Work out the finished part from the listing and answer in its coordinate system (mm). A direction names the side the tool comes from. Round coordinates to 2 decimals unless told otherwise and drop trailing zeros. Order: outer loops, then holes, each group sorted by start corner. A loop starts at its lowest first (then second) coordinate and runs counter-clockwise, first axis right, second up. Notation, with made-up numbers: (68, -18.75) - (72, -18.75) arc R26 ccw to (72, -3.75) - close; hole circle Ø3 at (38, 50). An arc over 180 degrees is marked (long way). Answer in a Markdown table with one row per item.
Autodesk Inventor part; units mm, degrees
ref_plane "Arbeitsebene2" through (4.7579, -7.132, 2.2) normal (0, 0, 1) x (1, 0, 0)
ref_plane "YZ Plane" through (0, 0, 0) normal (1, 0, 0) x (0, 1, 0)
ref_plane "XZ Plane" through (0, 0, 0) normal (0, 1, 0) x (-1, 0, 0)
ref_plane "Arbeitsebene1" through (0, 0, 0) normal (0, 0, 1) x (1, 0, 0)
sketch "Skizze1" plane through (0, 0, 0) normal (0, 0, 1) x (1, 0, 0)
  circle A0 centre (-0.0001, 0.0021) radius 3
  circle A1 centre (11, 0) radius 2.566
  circle A2 centre (-9.5, -11) radius 1.352
  arc A3 (19, -13.5) -> (20, -12.5) centre (19, -12.5) ccw
  line L0 (20, -12.5) -> (20, 12.5)
  arc A4 (20, 12.5) -> (19, 13.5) centre (19, 12.5) ccw
  line L1 (19, 13.5) -> (-19, 13.5)
  arc A5 (-19, 13.5) -> (-20, 12.5) centre (-19, 12.5) ccw
  line L2 (-20, 12.5) -> (-20, -12.5)
  arc A6 (-20, -12.5) -> (-19, -13.5) centre (-19, -12.5) ccw
  line L3 (-19, -13.5) -> (19, -13.5)
  line L4 (18.6579, -7.132) -> (11.0758, -7.132)
  line L5 (18.6579, -7.132) -> (18.6579, 2.268)
  line L6 (18.6579, 2.268) -> (19.6579, 4.268)
  line L7 (19.6579, 4.268) -> (19.6579, 7.668)
  line L8 (18.0704, 7.668) -> (19.6579, 7.668)
  line L9 (18.0704, 7.668) -> (18.0704, 6.818)
  line L10 (18.0704, 6.818) -> (13.4704, 6.818)
  line L11 (13.4704, 6.818) -> (13.4704, 5.418)
  line L12 (13.4704, 5.418) -> (14.8704, 5.418)
  line L13 (14.8704, 5.418) -> (15.4704, 6.018)
  line L14 (15.4704, 6.018) -> (18.0704, 6.018)
  line L15 (18.0704, 6.018) -> (18.0704, 5.768)
  line L16 (18.0704, 5.768) -> (15.5704, 5.768)
  line L17 (15.5704, 5.768) -> (15.0704, 5.268)
  line L18 (15.0704, 5.268) -> (13.0704, 5.268)
  line L19 (13.0704, 5.268) -> (13.0704, 7.668)
  line L20 (6.4079, 7.668) -> (13.0704, 7.668)
  line L21 (6.4079, 7.668) -> (6.4079, 6.468)
  line L22 (4.7579, 6.468) -> (6.4079, 6.468)
  line L23 (4.7579, -7.132) -> (4.7579, 6.468)
  line L24 (5.4458, -7.132) -> (4.7579, -7.132)
  line L25 (5.4458, -7.132) -> (5.4458, -6.382)
  line L26 (5.4458, -6.382) -> (11.0758, -6.382)
  line L27 (11.0758, -6.382) -> (11.0758, -7.132)
  line L28 (9.0327, 10.168) -> (-5.2421, 10.168)
  line L29 (-5.2421, 10.168) -> (-5.2421, 8.168)
  line L30 (-5.2421, 8.168) -> (9.0327, 8.168)
  line L31 (9.0327, 8.168) -> (9.0327, 10.168)
  line L32 (-5.2421, 8.168) -> (4.7579, 8.168)
  line L33 (4.7579, 8.168) -> (4.7579, -9.632)
  line L34 (4.7579, -9.632) -> (-5.2421, -9.632)
  line L35 (-5.2421, -9.632) -> (-5.2421, 8.168)
  line L36 (4.7579, -9.632) -> (9.0327, -9.632)
  line L37 (9.0327, -9.632) -> (9.0327, -7.632)
  line L38 (9.0327, -7.632) -> (4.7579, -7.632)
  line L39 (4.7579, -7.632) -> (4.7579, -9.632)
  point P0 (0, 0)
  point P1 (4.7579, 8.168)
  dimension "d0" = 0
  dimension "d1" = 0.5
  dimension "d2" = 0.5
  dimension "d3" = 2
  dimension "d4" = 2
  dimension "d5" = 10
ref_plane "Arbeitsebene2" through (4.7579, -7.132, 2.2) normal (0, 0, 1) x (1, 0, 0)
extrude "Extrusion1" add sketch "Skizze1" along normal up to surface (2.2 mm away) contours A0 | L33 L34 L35 L30 L23 | L38 L37 L36 L33 | L30 L29 L28 L31
sketch "Skizze2" plane through (-5.2421, 10.168, 2.2) normal (0, 0, 1) x (1, 0, 0)
  line L0 (0, 0) -> (14.2747, 0)
  line L1 (0, -19.8) -> (0, 0)
  line L2 (14.2747, -19.8) -> (0, -19.8)
  line L3 (14.2747, -17.8) -> (14.2747, -19.8)
  line L4 (10, -17.8) -> (14.2747, -17.8)
  line L5 (10, -2) -> (10, -17.8)
  line L6 (14.2747, -2) -> (10, -2)
  line L7 (14.2747, 0) -> (14.2747, -2)
  line L8 (14.2747, 0) -> (0, 0)
  line L9 (14.2747, 0) -> (0, 0)
  line L10 (0, 0) -> (0, -19.8)
  line L11 (0, -19.8) -> (14.2747, -19.8)
  line L12 (14.2747, -19.8) -> (14.2747, 0)
  line L13 (9.6421, -14.568) -> (0.8421, -14.568)
  line L14 (0.8421, -14.568) -> (0.8421, -5.768)
  line L15 (0.8421, -5.768) -> (9.6421, -5.768)
  line L16 (9.6421, -5.768) -> (9.6421, -14.568)
  line L17 (9.6421, -14.568) -> (0.8421, -5.768) construction
  line L18 (0.8421, -14.568) -> (9.6421, -5.768) construction
  line L19 (0, 0) -> (0, -19.8)
  line L20 (0.8421, -5.768) -> (0, -5.768)
  line L21 (0, -5.768) -> (0, -14.568)
  line L22 (0, -14.568) -> (0.8421, -14.568)
  line L23 (0.8421, -14.568) -> (0.8421, -5.768)
  point P0 (5.2421, -10.168)
  point P1 (0, -5.768)
  point P2 (0.8421, -14.568)
  point P3 (14.2747, -17.8)
  point P4 (14.2747, -2)
  dimension "d8" = 8.8
  dimension "d9" = 8.8
extrude "Extrusion2" add sketch "Skizze2" along normal blind 2 contours L0 L7 L6 L5 L4 L3 L2 L1 L22 L13 L16 L15 L20 | L12 L4 L5 L6
sketch "Skizze3" plane through (0, 0, 0) normal (0, 0, -1) x (-1, 0, 0)
  line L0 (5.2421, 10.168) -> (5.2421, -9.632)
  line L1 (-9.0327, 10.168) -> (5.2421, 10.168)
  line L2 (-9.0327, 8.168) -> (-9.0327, 10.168)
  line L3 (-4.7579, 8.168) -> (-9.0327, 8.168)
  line L4 (-4.7579, -7.632) -> (-4.7579, 8.168)
  line L5 (-9.0327, -7.632) -> (-4.7579, -7.632)
  line L6 (-9.0327, -9.632) -> (-9.0327, -7.632)
  line L7 (5.2421, -9.632) -> (-9.0327, -9.632)
  line L8 (2.2421, -9.8367) -> (9.0217, -9.8367)
  line L9 (9.0217, -9.8367) -> (9.0217, 10.4786)
  line L10 (9.0217, 10.4786) -> (2.2421, 10.4786)
  line L11 (2.2421, 10.4786) -> (2.2421, -9.8367)
  line L12 (2.2421, -9.8367) -> (9.0217, 10.4786) construction
  line L13 (9.0217, -9.8367) -> (2.2421, 10.4786) construction
  point P0 (0, 0)
  point P1 (5.6319, 0.321)
  dimension "d12" = 3
extrude "Extrusion3" cut sketch "Skizze3" against normal blind 2.5 contours L1 L11 L10 L9 L8 L7 L0 | L0 L7 L11 L1
sketch "Skizze4" plane through (0, 0, 0) normal (0, 0, -1) x (-1, 0, 0)
  line L0 (2.2421, -9.632) -> (2.2421, 10.168)
  line L1 (-9.0327, 10.168) -> (2.2421, 10.168)
  line L2 (-9.0327, 8.168) -> (-9.0327, 10.168)
  line L3 (-4.7579, 8.168) -> (-9.0327, 8.168)
  line L4 (-4.7579, -7.632) -> (-4.7579, 8.168)
  line L5 (-9.0327, -7.632) -> (-4.7579, -7.632)
  line L6 (-9.0327, -9.632) -> (-9.0327, -7.632)
  line L7 (2.2421, -9.632) -> (-9.0327, -9.632)
  line L8 (2.2421, 4.4) -> (2.2421, 10.168)
  line L9 (2.2421, 9.168) -> (-1.1963, 9.168)
  line L10 (-1.1963, 9.168) -> (-1.1963, -8.632)
  line L11 (-1.1963, -8.632) -> (2.2421, -8.632)
  line L12 (2.2421, -8.632) -> (2.2421, 9.168)
  point P0 (0, 0)
  point P1 (2.2421, -8.632)
extrude "Extrusion4" cut sketch "Skizze4" against normal blind 2 contours L11 L10 L9 L0
equation "\"d6\" = d2"
properties part number "Anglerfish_Cameraspacer"
1) Find section D-D, the plane x = 5.5. Give the vertices of the cut face in (y, z).
Filled in:
| item | result |
|---|---|
| outline | (-9.63, 0) - (-7.63, 0) - (-7.63, 2.2) - (8.17, 2.2) - (8.17, 0) - (10.17, 0) - (10.17, 4.2) - (-9.63, 4.2) - close |
2) Find the intervals of material crossed by probe 1 along Y at (x, z) = (5.5, 1.65); probe 2 along Y at (x, z) = (-1.75, 1.9); probe 3 along Z at (x, y) = (-4.25, 8.75), in increasing order. Write a range as from..to.
Filled in:
| item | result |
|---|---|
| probe 1 | y = -9.63..-7.63, 8.17..10.17 |
| probe 2 | y = -9.63..-8.63, 9.17..10.17 |
| probe 3 | z = 2.5..4.2 |
3) Find section B-B, the plane y = -0.25. Give the vertices of the cut face in (x, z), then the cut area to 3 significant figures.
Filled in:
| item | result |
|---|---|
| outline | (-2.24, 2) - (1.2, 2) - (1.2, 0) - (4.76, 0) - (4.76, 2.2) - (9.03, 2.2) - (9.03, 4.2) - (4.4, 4.2) - (4.4, 2.2) - (-2.24, 2.2) - close |
| area | 17.8 mm^2 |
4) Each of these flat-tipped pins is pushed along its axis until it touches: pin 1 (3.5 mm diameter, centred on x = 7, y = 1.5, fed in from -Z); pin 2 (0.6 mm diameter, centred on y = 2.5, z = 0.5, fed in from -X); pin 3 (0.8 mm diameter, centred on y = -2, z = 2, fed in from -X). Where does it stop, or does it pass through?
Filled in:
| item | result |
|---|---|
| pin 1 | stops at z = 2.2 |
| pin 2 | stops at x = 1.2 |
| pin 3 | stops at x = -2.24 |
5) Find section A-A, the plane x = -3.75. Give the vertices of the cut face in (y, z), then the cut area to 3 significant figures.
Filled in:
| item | result |
|---|---|
| outline | (-9.63, 2.5) - (-4.4, 2.5) - (-4.4, 4.2) - (-9.63, 4.2) - close; (4.4, 2.5) - (10.17, 2.5) - (10.17, 4.2) - (4.4, 4.2) - close |
| area | 18.7 mm^2 |
6) Which of the six approach directions +Z, -Z, +X, -X, +Y, -Y give full straight-line access (tool end or side, diameter ignored) to faces 1 (the face through (-1, 9.168, 1)), 2 (the face through (4.758, 0, 1)), 3 (the face through (2, -9.632, 2)), 4 (the face through (-4, -7, 2.5)), 5 (the face through (1, 0, 2.2))?
Filled in:
| item | result |
|---|---|
| face 1 | -Z, -X |
| face 2 | -Z, +X |
| face 3 | +Z, -Z, +X, -X, -Y |
| face 4 | -Z, -X, +Y, -Y |
| face 5 | +Z, -X |
7) Find section C-C, the plane z = 0.4. Give the vertices of the cut face in (x, y).
Filled in:
| item | result |
|---|---|
| outline | (-2.24, -9.63) - (9.03, -9.63) - (9.03, -7.63) - (4.76, -7.63) - (4.76, 8.17) - (9.03, 8.17) - (9.03, 10.17) - (-2.24, 10.17) - (-2.24, 9.17) - (1.2, 9.17) - (1.2, -8.63) - (-2.24, -8.63) - close |
8) The mould has two halves that part along Y. Classify faces 6 (the face through (0, -4.4, 3)), 7 (the face through (5, 0, 4.2)), 8 (the face through (2, 10.168, 2)): released by +Y, released by -Y, zero draft, split by the parting line, or undercut.
Filled in:
| item | result |
|---|---|
| face 6 | undercut |
| face 7 | zero draft |
| face 8 | released by +Y |
